```python
from build123d import *

# Parameters (mm, degrees)
SKETCH3_W           = 101
SKETCH3_H           = 22
SKETCH3_W_2         = 14
SKETCH3_H_2         = 14
SKETCH3_W_3         = 13.9
SKETCH3_H_3         = 13.9
SKETCH3_W_4         = 13.8
SKETCH3_H_4         = 13.8
SKETCH3_W_5         = 13.7
SKETCH3_H_5         = 13.7
BOSS_EXTRUDE5_DEPTH = 4.5


with BuildPart() as part:
    # Sketch3 → Boss-Extrude5 (new body)
    with BuildSketch(Plane(origin=(0, 0, 0), x_dir=(1, 0, 0), z_dir=(0, 1, 0))):
        with Locations((50.5, 11)):
            Rectangle(SKETCH3_W, SKETCH3_H)
        with Locations((13, 11)):
            Rectangle(SKETCH3_W_2, SKETCH3_H_2, mode=Mode.SUBTRACT)
        with Locations((38, 11)):
            Rectangle(SKETCH3_W_3, SKETCH3_H_3, mode=Mode.SUBTRACT)
        with Locations((63, 11)):
            Rectangle(SKETCH3_W_4, SKETCH3_H_4, mode=Mode.SUBTRACT)
        with Locations((88, 11)):
            Rectangle(SKETCH3_W_5, SKETCH3_H_5, mode=Mode.SUBTRACT)
    extrude(amount=BOSS_EXTRUDE5_DEPTH)


solid = part.part
```
Work out the finished part from the listing and answer in its coordinate system (mm). A direction names the side the tool comes from. Round coordinates to 2 decimals unless told otherwise and drop trailing zeros. Loops run counter-clockwise (first coordinate to the right, second up) from the corner with the lowest first, then second, coordinate; pieces in that order, holes last. Notation, with made-up numbers: (8.5, 80.25) -> (24.5, 80.25) arc R36 cw to (24.5, 115.25) -> close; hole circle Ø10 at (83.25, -15). An arc over 180 degrees is marked (long way). Write each question's results on one line, items separated by ' | '. Start each with the question number.
1. Section C-C (y = 3.35) is taken. Determine the outline of the cut face in (x, z), plus the area to 3 significant figures.
2. Section D-D (x = 87) is taken. Determine the outline of the cut face in (y, z).
3. Given pin 1 Ø1.3 at (x, y) = (11, 2.5) entering from +Z, flat-ended and moving along its own axis, determine where the tip first touches the part or whether it passes through.
4. Section B-B (x = 60.5) is taken. Determine the outline of the cut face in (y, z), plus the area to 3 significant figures.
5. Find the intervals of material crossed by probe 1 along X at (y, z) = (0.35, -11.5); probe 2 along Z at (x, y) = (60, 2.35); probe 3 along Z at (x, y) = (16, 3.3), in increasing order. Write a range as from..to.
6. A tool of negligible diameter and unlimited length cuts with its end or side. For faces 1 (the face through (20, 2, -11)), 2 (the face through (50, 2, 0)), from which of +Z, -Z, +X, -X, +Y, -Y can it reach the whole face along a straight path? Write none if from no direction.
7. For a pull along X with two mould halves and no side action, classify faces 3 (the face through (63, 2, -4.1)), 4 (the face through (0, 2, -11)), 5 (the face through (50, 2, -22)) as +X half, -X half, draft (parallel to the pull), parting line (faces both ways), or undercut.
8. Section A-A (z = -8) is taken. Determine the outline of the cut face in (x, y).
Evaluation:
1) outline: (0, -22) -> (101, -22) -> (101, 0) -> (0, 0) -> close; hole (6, -18) -> (20, -18) -> (20, -4) -> (6, -4) -> close; hole (31.05, -17.95) -> (44.95, -17.95) -> (44.95, -4.05) -> (31.05, -4.05) -> close; hole (56.1, -17.9) -> (69.9, -17.9) -> (69.9, -4.1) -> (56.1, -4.1) -> close; hole (81.15, -17.85) -> (94.85, -17.85) -> (94.85, -4.15) -> (81.15, -4.15) -> close | area: 1,450 mm2
2) outline: (0, -22) -> (4.5, -22) -> (4.5, -17.85) -> (0, -17.85) -> close; (0, -4.15) -> (4.5, -4.15) -> (4.5, 0) -> (0, 0) -> close
3) pin 1: stops at z = 0
4) outline: (0, -22) -> (4.5, -22) -> (4.5, -17.9) -> (0, -17.9) -> close; (0, -4.1) -> (4.5, -4.1) -> (4.5, 0) -> (0, 0) -> close | area: 36.9 mm2
5) probe 1: x = 0..6, 20..31.05, 44.95..56.1, 69.9..81.15, 94.85..101 | probe 2: z = -22..-17.9, -4.1..0 | probe 3: z = -22..-18, -4..0
6) face 1: +Y, -Y | face 2: +Z, +X, -X, +Y, -Y
7) face 3: undercut | face 4: -X half | face 5: draft
8) outline: (0, 0) -> (6, 0) -> (6, 4.5) -> (0, 4.5) -> close; (20, 0) -> (31.05, 0) -> (31.05, 4.5) -> (20, 4.5) -> close; (44.95, 0) -> (56.1, 0) -> (56.1, 4.5) -> (44.95, 4.5) -> close; (69.9, 0) -> (81.15, 0) -> (81.15, 4.5) -> (69.9, 4.5) -> close; (94.85, 0) -> (101, 0) -> (101, 4.5) -> (94.85, 4.5) -> close
